```python
from build123d import *

# Parameters (mm, degrees)
F1_DEPTH = 6


with BuildPart() as f1:
    # F0 (on Front) → F1 (new body)
    with BuildSketch(Plane.XZ):
        with BuildLine():
            Line((-113.7830221973, 196.5653101416), (-116.9823558728, 146.4273122476))
            add(Edge.make_bspline(
                [(-116.9823558728, 146.4273122476), (-91.5295582515, 161.7084143763), (-84.4563773973, 172.3099058233), (-56.413200461, 181.8094376312)],
                knots=[0.6217299922, 0.6217299922, 0.6217299922, 0.6217299922, 1, 1, 1, 1], degree=3))
            ThreePointArc((-56.413200461, 181.8094376312), (35.1094960363, 186.4278723491), (116.4179808184, 144.1589213822))
            Line((116.4179808184, 144.1589213822), (-28.0945999151, 310.6102859554))
            Line((-28.0945999151, 310.6102859554), (-31.1034692521, 310.5229280694))
            Line((-31.1034692521, 310.5229280694), (-53.0575460655, 232.5305113428))
            ThreePointArc((-53.0575460655, 232.5305113428), (-71.8460560006, 205.592638023), (-103.2941289159, 196.1229054773))
            Line((-103.2941289159, 196.1229054773), (-113.7830221973, 196.5653101416))
        make_face()
    extrude(amount=F1_DEPTH)


solid = f1.part
```
Read the model definition and answer for the solid it produces. Units are mm, in the model's axes. A direction names the side the tool comes from. Coordinates: 2 decimals unless noted, no trailing zeros. Write each loop counter-clockwise with the first axis right and the second up, starting at its lowest first coordinate (ties: lowest second). Pieces come first, ordered by that corner, then holes. Notation, with made-up numbers: (-20, 38) - (0, 38) arc R35 ccw to (0, 75) - close; hole circle Ø7 at (-20, 1.5). An arc over 180 degrees is marked (long way). Answer as a JSON object with one key per item and string values. Group by question number.
1. Consider L1, parallel to X at y = -2.5, z = 177; L2, parallel to Z at x = 5, y = -0.25; L3, parallel to Z at x = -23, y = -1.5. Determine where each line is inside the solid, lowest interval first. Write a range as [from, to].
2. The mould has two halves that part along X. Classify faces 3 (the flat face through (-18, -6, 222)), 4 (the flat face through (-115.36, -2.96, 171.85)), 5 (the cylindrical face through (33.84, -2.96, 186.7)): +X half, -X half, draft (parallel to the pull), parting line (faces both ways), or undercut.
3. A cutting plane is placed at A-A (z = 186). Determine the outline of the cut face in (x, y), plus the area to 3 significant figures.
4. A cutting plane is placed at B-B (x = -40). Determine the outline of the cut face in (y, z), plus the area to 3 significant figures.
5. Which of the six approach directions +Z, -Z, +X, -X, +Y, -Y give full straight-line access (tool end or side, diameter ignored) to faces 1 (the flat face through (-108.47, -2.96, 196.34)), 2 (the flat face through (-41.927, -2.958, 272.073))?
6. A cutting plane is placed at C-C (z = 252). Determine the outline of the cut face in (x, y), plus the area to 3 significant figures.
7. Each of these flat-tipped pins is pushed along its axis until it touches: P1, Ø2, axis at x = -1, y = -3, coming from the +Z side; P2, Ø1, axis at y = -2.5, z = 167.5, coming from the +X side; P3, Ø2, axis at x = -40, y = -2, coming from the -Z side. Where does it stop, or does it pass through?
Worked out:
{
 "1": {"L1": "x = [-115.03, -68.76], [65.11, 87.91]", "L2": "z = [190.29, 272.49]", "L3": "z = [189.19, 304.74]"},
 "2": {"face 3": "draft", "face 4": "-X half", "face 5": "undercut"},
 "3": {"outline": "(-114.46, -6) - (-41.3, -6) - (-41.3, 0) - (-114.46, 0) - close; (37.02, -6) - (80.09, -6) - (80.09, 0) - (37.02, 0) - close", "area": "697 mm²"},
 "4": {"outline": "(-6, 186.29) - (0, 186.29) - (0, 278.92) - (-6, 278.92) - close", "area": "556 mm²"},
 "5": {"face 1": "+Z, +Y, -Y", "face 2": "+Z, -X, +Y, -Y"},
 "6": {"outline": "(-47.58, -6) - (22.79, -6) - (22.79, 0) - (-47.58, 0) - close", "area": "422 mm²"},
 "7": {"P1": "stops at z = 280.55", "P2": "stops at x = 96.59", "P3": "stops at z = 186.07"}
}
